The model under review builds one solid part; all positions refer to its coordinate system, in mm. Face numbers are marked on the shaded views. A direction names the side the tool comes from. Round coordinates to 2 decimals unless told otherwise and drop trailing zeros. Order: outer loops, then holes, each group sorted by start corner. A loop starts at its lowest first (then second) coordinate and runs counter-clockwise, first axis right, second up. Notation, with made-up numbers: M -35,34.5 L 4,34.5 A21 ccw 4,70.5 Z; hole C -22.75,-4 d9. An arc over 180 degrees is marked long. One line per item, written item: value. Start each with the question number.
from build123d import *

# Parameters (mm, degrees)
EXTRUDE_THIN1_DEPTH     = 101.6
FILLET1_R               = 25.4
FILLET2_R               = 25.4
CUT_EXTRUDE1_DEPTH      = 10.922
CUT_EXTRUDE1_DEPTH_BACK = 54.61
CUT_EXTRUDE2_DEPTH      = 14.224
CUT_EXTRUDE2_DEPTH_BACK = 17.78
SKETCH4_R               = 1.5875
CUT_EXTRUDE3_DEPTH      = 14.732
CUT_EXTRUDE3_DEPTH_BACK = 23.876
SKETCH5_R               = 1.5875
CUT_EXTRUDE5_DEPTH      = 15.24
CUT_EXTRUDE5_DEPTH_BACK = 39.37
SKETCH6_R               = 1.5875


with BuildPart() as part:
    # Sketch1 → Extrude-Thin1 (new, symmetric)
    with BuildSketch(Plane.XY):
        with BuildLine():
            Line((0, 0), (0, 5.08))
            ThreePointArc((0, 5.08), (-3.719743879, 14.060256121), (-12.7, 17.78))
            ThreePointArc((-12.7, 17.78), (-30.660512242, 25.219487758), (-38.1, 43.18))
            Line((-38.1, 43.18), (-38.1, 360.68))
            Line((-38.1, 360.68), (-30.48, 360.68))
            Line((-30.48, 360.68), (-30.48, 43.18))
            ThreePointArc((-30.48, 43.18), (-25.272358569, 30.607641431), (-12.7, 25.4))
            ThreePointArc((-12.7, 25.4), (1.668409794, 19.448409794), (7.62, 5.08))
            Line((7.62, 5.08), (7.62, 0))
            Line((7.62, 0), (0, 0))
        make_face()
    extrude(amount=EXTRUDE_THIN1_DEPTH, both=True)

    # Fillet1
    fillet1_edges = [part.edges().sort_by_distance(p)[0] for p in [
        (-34.29, 360.68, 101.6),
    ]]
    fillet(fillet1_edges, radius=FILLET1_R)

    # Fillet2
    fillet2_edges = [part.edges().sort_by_distance(p)[0] for p in [
        (-34.29, 360.68, -101.6),
    ]]
    fillet(fillet2_edges, radius=FILLET2_R)

    # Sketch3 → Cut-Extrude1 (cut, two sides: drawn at the far end of the back side and taken through both)
    with BuildSketch(Plane(origin=(7.62, 0, 0), x_dir=(0, 0, -1), z_dir=(1, 0, 0)).offset(-CUT_EXTRUDE1_DEPTH_BACK)):
        with BuildLine():
            Line((-101.6, 0), (-101.6, 63.533291796))
            ThreePointArc((-101.6, 63.533291796), (-82.785279567, 34.211252412), (-76.2, 0))
            Line((-76.2, 0), (-101.6, 0))
        make_face()
        with BuildLine():
            Line((101.6, 0), (76.2, 0))
            ThreePointArc((76.2, 0), (82.785279567, 34.211252412), (101.6, 63.533291796))
            Line((101.6, 63.533291796), (101.6, 0))
        make_face()
    extrude(amount=CUT_EXTRUDE1_DEPTH + CUT_EXTRUDE1_DEPTH_BACK, mode=Mode.SUBTRACT)

    # Sketch4 → Cut-Extrude2 (cut, two sides: drawn at the far end of the back side and taken through both)
    with BuildSketch(Plane(origin=(-30.48, 0, 0), x_dir=(0, 0, -1), z_dir=(1, 0, 0)).offset(-CUT_EXTRUDE2_DEPTH_BACK)):
        with Locations(Location((-89.003908419, 284.48, 0), (0, 0, 180))):
            Circle(SKETCH4_R)
        with Locations(Location((88.803751124, 284.48, 0), (0, 0, 180))):
            Circle(SKETCH4_R)
    extrude(amount=CUT_EXTRUDE2_DEPTH + CUT_EXTRUDE2_DEPTH_BACK, mode=Mode.SUBTRACT)

    # Sketch5 → Cut-Extrude3 (cut, two sides: drawn at the far end of the back side and taken through both)
    with BuildSketch(Plane(origin=(0, 25.4, 0), x_dir=(1, 0, 0), z_dir=(0, 1, 0)).offset(-CUT_EXTRUDE3_DEPTH_BACK)):
        with Locations(Location((-12.7, -60.719407292, 0), (0, 0, 90))):
            Circle(SKETCH5_R)
        with Locations(Location((-12.7, 60.719407292, 0), (0, 0, 90))):
            Circle(SKETCH5_R)
    extrude(amount=CUT_EXTRUDE3_DEPTH + CUT_EXTRUDE3_DEPTH_BACK, mode=Mode.SUBTRACT)

    # Sketch6 → Cut-Extrude5 (cut, two sides: drawn at the far end of the back side and taken through both)
    with BuildSketch(Plane(origin=(7.62, 0, 0), x_dir=(0, 0, -1), z_dir=(1, 0, 0)).offset(-CUT_EXTRUDE5_DEPTH_BACK)):
        with Locations(Location((-50.940117855, 5.08, 0), (0, 0, 180))):
            Circle(SKETCH6_R)
        with Locations(Location((50.940117855, 5.08, 0), (0, 0, 180))):
            Circle(SKETCH6_R)
    extrude(amount=CUT_EXTRUDE5_DEPTH + CUT_EXTRUDE5_DEPTH_BACK, mode=Mode.SUBTRACT)


solid = part.part
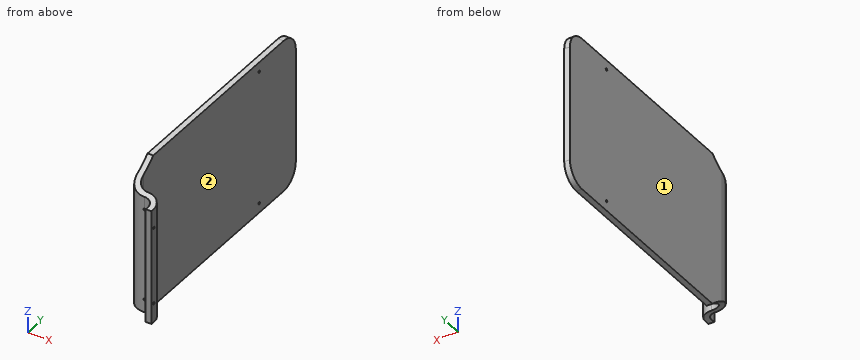
Item 1: Consider section A-A, the plane z = -12. Give the boundary of the cut face in (x, y), then the cut area to 3 significant figures.
Item 2: Consider section B-B, the plane y = 246. Give the boundary of the cut face in (x, z).
Item 3: Consider section C-C, the plane x = -21. Give the boundary of the cut face in (y, z), then the cut area to 3 significant figures.
Item 4: Machinability: for the marked faces 1 and 2, which of the approach directions +Z, -Z, +X, -X, +Y, -Y give a long, thin tool a straight path to every point of the face, cutting with its end or side? Answer none if there is none.
Item 5: Clearance check with flat-ended pins moving along their axes: P1, Ø5.5, axis at y = 3, z = 1.5, coming from the -X side; P2, Ø1.9, axis at y = 284.48, z = -88.8, coming from the -X side; P3, Ø4, axis at y = 5.08, z = 50.94, coming from the -X side; P4, Ø5, axis at y = 284.48, z = 89, coming from the +X side. State where each tip first meets the part, or that it passes through.
Item 6: Wall thickness on L1, parallel to Z at x = 1.5, y = 5.08; L2, parallel to Z at x = -12.7, y = 21.5; L3, parallel to X at y = 233, z = 88: over which ranges is each line inside the solid? List them lowest first.
Computed:
1. outline: M -38.1,43.18 A25.4 ccw -12.7,17.78 A12.7 cw 0,5.08 L 0,0 L 7.62,0 L 7.62,5.08 A20.32 ccw -12.7,25.4 A17.78 cw -30.48,43.18 L -30.48,360.68 L -38.1,360.68 Z
1. area: 2,910 mm^2
2. outline: M -38.1,-101.6 L -30.48,-101.6 L -30.48,101.6 L -38.1,101.6 Z
3. outline: M 19.17,-78.22 A92.16 cw 27.46,-80.38 L 27.46,80.38 A92.16 cw 19.17,78.22 Z
3. area: 1,310 mm^2
4. face 1: +Z, -Z, -X, +Y, -Y
4. face 2: +Z, -Z, +X, +Y
5. P1: stops at x = -0.02
5. P2: passes through
5. P3: stops at x = -0.16
5. P4: stops at x = -30.48
6. L1: z = -76.34 to -52.53, -49.35 to 49.35, 52.53 to 76.34
6. L2: z = -78.74 to -62.31, -59.13 to 59.13, 62.31 to 78.74
6. L3: x = -38.1 to -30.48
